CAD build for the part. Positions are in the model's coordinates, mm. A direction names the side the tool comes from. Give positions to 0.01 mm unless a question says otherwise; leave off trailing zeros. Loops run counter-clockwise (first coordinate to the right, second up) from the corner with the lowest first, then second, coordinate; pieces in that order, holes last.
```python
from build123d import *

# Parameters (mm, degrees)
SKETCH1_W           = 160
SKETCH1_H           = 95
BOSS_EXTRUDE1_DEPTH = 15
SHELL1_T            = -2.5
SKETCH2_W           = 21
SKETCH2_H           = 13
CUT_EXTRUDE1_DEPTH  = 15
FILLET2_R           = 2
FILLET8_R           = 2
FILLET13_R          = 2


with BuildPart() as part:
    # Sketch1 → Boss-Extrude1 (new body)
    with BuildSketch(Plane(origin=(0, 0, 0), x_dir=(1, 0, 0), z_dir=(0, 1, 0))):
        with Locations((5.685950413, -3.070247934)):
            Rectangle(SKETCH1_W, SKETCH1_H)
    extrude(amount=BOSS_EXTRUDE1_DEPTH)

    # Shell1
    shell1_openings = [part.faces().sort_by_distance(p)[0] for p in [
        (5.685950413, 15, 3.070247934),
    ]]
    offset(amount=SHELL1_T, openings=shell1_openings, kind=Kind.INTERSECTION)

    # Sketch2 → Cut-Extrude1 (cut)
    with BuildSketch(Plane(origin=(0, 0, 0), x_dir=(1, 0, 0), z_dir=(0, 1, 0))):
        with Locations((-52.103761913, -32.277000916)):
            Rectangle(SKETCH2_W, SKETCH2_H)
    extrude(amount=CUT_EXTRUDE1_DEPTH, mode=Mode.SUBTRACT)

    # Fillet2
    fillet2_edges = [part.edges().sort_by_distance(p)[0] for p in [
        (5.685950413, 15, -44.429752066),
        (-74.314049587, 15, 3.070247934),
        (5.685950413, 0, -44.429752066),
        (85.685950413, 0, 3.070247934),
        (5.685950413, 0, 50.570247934),
        (-74.314049587, 0, 3.070247934),
        (-74.314049587, 7.5, -44.429752066),
        (85.685950413, 7.5, -44.429752066),
        (-74.314049587, 7.5, 50.570247934),
    ]]
    fillet(fillet2_edges, radius=FILLET2_R)

    # Fillet8
    # the kernel refuses this fillet: 2 mm, written as the material it adds along each edge
    with BuildSketch(Plane(origin=(-71.814049587, 2.5, -41.929752066), x_dir=(0, 1, 0), z_dir=(0, 0, 1))) as fillet8_piece_1:
        with BuildLine():
            CenterArc((FILLET8_R, -FILLET8_R), FILLET8_R, 90, 90)
            Line((0, -FILLET8_R), (0, 0))
            Line((0, 0), (FILLET8_R, 0))
        make_face()
    extrude(amount=90)
    # the kernel refuses this fillet: 2 mm, written as the material it takes off along each edge
    with BuildSketch(Plane(origin=(83.685950413, 13, -42.429752066), x_dir=(1, 0, 0), z_dir=(0, 1, 0))) as fillet8_2_piece_1_section:
        Polygon((0, 0), (FILLET8_R * 1.02, 0), (FILLET8_R * 1.02, FILLET8_R * 1.02), (0, FILLET8_R * 1.02), align=None)
    fillet8_2_piece_1 = extrude(amount=FILLET8_R * 1.02, mode=Mode.PRIVATE)
    fillet8_2_piece_1 = fillet8_2_piece_1 - Plane(origin=(83.685950413, 13, -42.429752066), x_dir=(-0.7071067811865476, 0, 0.7071067811865475), z_dir=(0, 1, 0)) * Sphere(FILLET8_R, mode=Mode.PRIVATE)
    add(fillet8_2_piece_1, mode=Mode.SUBTRACT)
    with BuildSketch(Plane(origin=(83.685950413, 2, 48.570247934), x_dir=(0, 0, 1), z_dir=(1, 0, 0))) as fillet8_2_piece_2_section:
        Polygon((0, 0), (FILLET8_R * 1.02, 0), (FILLET8_R * 1.02, FILLET8_R * 1.02), (0, FILLET8_R * 1.02), align=None)
    fillet8_2_piece_2 = extrude(amount=FILLET8_R * 1.02, mode=Mode.PRIVATE)
    fillet8_2_piece_2 = fillet8_2_piece_2 - Plane(origin=(83.685950413, 2, 48.570247934), x_dir=(0, 0.7071067811865475, -0.7071067811865475), z_dir=(1, 0, 0)) * Sphere(FILLET8_R, mode=Mode.PRIVATE)
    add(fillet8_2_piece_2, mode=Mode.SUBTRACT)
    with BuildSketch(Plane(origin=(-72.314049587, 13, 48.570247934), x_dir=(0, 0, 1), z_dir=(0, 1, 0))) as fillet8_2_piece_3_section:
        Polygon((0, 0), (FILLET8_R * 1.02, 0), (FILLET8_R * 1.02, -FILLET8_R * 1.02), (0, -FILLET8_R * 1.02), align=None)
    fillet8_2_piece_3 = extrude(amount=FILLET8_R * 1.02, mode=Mode.PRIVATE)
    fillet8_2_piece_3 = fillet8_2_piece_3 - Plane(origin=(-72.314049587, 13, 48.570247934), x_dir=(0.7071067811865475, 0, -0.7071067811865475), z_dir=(0, 1, 0)) * Sphere(FILLET8_R, mode=Mode.PRIVATE)
    add(fillet8_2_piece_3, mode=Mode.SUBTRACT)
    with BuildSketch(Plane(origin=(83.685950413, 13, 48.570247934), x_dir=(0, 0, 1), z_dir=(1, 0, 0))) as fillet8_2_piece_4_section:
        Polygon((0, 0), (FILLET8_R * 1.02, 0), (FILLET8_R * 1.02, -FILLET8_R * 1.02), (0, -FILLET8_R * 1.02), align=None)
    fillet8_2_piece_4 = extrude(amount=FILLET8_R * 1.02, mode=Mode.PRIVATE)
    fillet8_2_piece_4 = fillet8_2_piece_4 - Plane(origin=(83.685950413, 13, 48.570247934), x_dir=(0, -0.7071067811865475, -0.7071067811865475), z_dir=(1, 0, 0)) * Sphere(FILLET8_R, mode=Mode.PRIVATE)
    add(fillet8_2_piece_4, mode=Mode.SUBTRACT)
    with BuildSketch(Plane(origin=(85.685950413, 15, -42.429752066), x_dir=(-1, 0, 0), z_dir=(0, 0, 1))) as fillet8_2_piece_5:
        with BuildLine():
            CenterArc((FILLET8_R, FILLET8_R), FILLET8_R, 180, 90)
            Line((0, FILLET8_R), (0, 0))
            Line((0, 0), (FILLET8_R, 0))
        make_face()
    extrude(amount=91, mode=Mode.SUBTRACT)
    with BuildSketch(Plane(origin=(83.685950413, 15, 50.570247934), x_dir=(0, 0, -1), z_dir=(-1, 0, 0))) as fillet8_2_piece_6:
        with BuildLine():
            CenterArc((FILLET8_R, FILLET8_R), FILLET8_R, 180, 90)
            Line((0, FILLET8_R), (0, 0))
            Line((0, 0), (FILLET8_R, 0))
        make_face()
    extrude(amount=156, mode=Mode.SUBTRACT)
    with BuildSketch(Plane(origin=(85.685950413, 2, 50.570247934), x_dir=(0, 0, -1), z_dir=(0, 1, 0))) as fillet8_2_piece_7:
        with BuildLine():
            CenterArc((FILLET8_R, FILLET8_R), FILLET8_R, 180, 90)
            Line((0, FILLET8_R), (0, 0))
            Line((0, 0), (FILLET8_R, 0))
        make_face()
    extrude(amount=11, mode=Mode.SUBTRACT)

    # Fillet13
    fillet13_edges = [part.edges().sort_by_distance(p)[0] for p in [
        (-71.814049587, 9.75, 48.070247934),
        (83.185950413, 2.5, 3.070247934),
        (83.185950413, 8.75, 48.070247934),
        (6.685950413, 2.5, 48.070247934),
        (-71.228263149, 3.085786438, 48.070247934),
    ]]
    fillet(fillet13_edges, radius=FILLET13_R)


solid = part.part
```
1. Saw through at B-B, the plane x = -19.5. List the corners of the cut face in (y, z), and give its area (3 significant figures).
Responses:
outline: (0, -42.43) arc R2 ccw to (2, -44.43) - (13, -44.43) arc R2 ccw to (15, -42.43) - (15, -41.93) - (2.5, -41.93) - (2.5, 46.07) arc R2 cw to (4.5, 48.07) - (15, 48.07) - (15, 48.57) arc R2 ccw to (13, 50.57) - (2, 50.57) arc R2 ccw to (0, 48.57) - close
area: 297 mm2
2. Drop a flat-ended pin along its axis: pin 1 (1 mm diameter, centred on x = 16, z = -12, fed in from +Y). Give the stop position or say it passes through.
Responses:
pin 1: stops at y = 2.5
3. Pull direction Z, two halves, no side cores. Call faces 1 (the face through (5, 0, 2)), 2 (the face through (5, 2.5, 1)), 3 (the face through (5, 7, 50.57)), 4 (the face through (-71.814, 10, 3)): released by +Z, released by -Z, zero draft, split by the parting line, or undercut.
Responses:
face 1: zero draft
face 2: undercut
face 3: released by +Z
face 4: undercut
4. Saw through at C-C, the plane y = 6. List the corners of the cut face in (x, z), and give its area (3 significant figures).
Responses:
outline: (-74.31, -42.43) arc R2 ccw to (-72.31, -44.43) - (83.69, -44.43) arc R2 ccw to (85.69, -42.43) - (85.69, 48.57) arc R2 ccw to (83.69, 50.57) - (-72.31, 50.57) arc R2 ccw to (-74.31, 48.57) - close; hole (-71.81, -41.93) - (83.19, -41.93) - (83.19, 46.07) arc R2 ccw to (81.19, 48.07) - (-69.81, 48.07) arc R2 ccw to (-71.81, 46.07) - close
area: 1,250 mm2
5. Probe line 1 along Z through (x, y) = (8.5, 7.75); line 2 along X through (y, z) = (6.5, 12.5); line 3 along Y through (x, z) = (28, 6). List the from-to ranges inside material, lowest first.
Responses:
line 1: z = -44.43 to -41.93, 48.07 to 50.57
line 2: x = -74.31 to -71.81, 83.19 to 85.69
line 3: y = 0 to 2.5
6. Saw through at D-D, the plane z = 0. List the corners of the cut face in (x, y), and give its area (3 significant figures).
Responses:
outline: (-74.31, 2) arc R2 ccw to (-72.31, 0) - (83.69, 0) arc R2 ccw to (85.69, 2) - (85.69, 13) arc R2 ccw to (83.69, 15) - (83.19, 15) - (83.19, 4.5) arc R2 cw to (81.19, 2.5) - (-69.81, 2.5) arc R2 cw to (-71.81, 4.5) - (-71.81, 15) - (-72.31, 15) arc R2 ccw to (-74.31, 13) - close
area: 461 mm2
7. Tool access for faces 5 (the face through (-74.314, 7, 4)), 6 (the face through (5, 10, 48.07)): list every direction of +Z, -Z, +X, -X, +Y, -Y with a clear straight run to the whole face (end or side of a thin tool).
Responses:
face 5: +Z, -Z, -X, +Y, -Y
face 6: +Y
8. Saw through at A-A, the plane z = 33.5. List the corners of the cut face in (x, y).
Responses:
outline: (-74.31, 2) arc R2 ccw to (-72.31, 0) - (-62.6, 0) - (-62.6, 2.5) - (-69.81, 2.5) arc R2 cw to (-71.81, 4.5) - (-71.81, 15) - (-72.31, 15) arc R2 ccw to (-74.31, 13) - close; (-41.6, 0) - (83.69, 0) arc R2 ccw to (85.69, 2) - (85.69, 13) arc R2 ccw to (83.69, 15) - (83.19, 15) - (83.19, 4.5) arc R2 cw to (81.19, 2.5) - (-41.6, 2.5) - close
